from build123d import *

# Parameters (mm, degrees)
BOSS_EXTRUDE1_DEPTH = 10
SKETCH2_R           = 1
BOSS_EXTRUDE2_DEPTH = 2.25


with BuildPart() as part:
    # Sketch1 → Boss-Extrude1 (new body)
    with BuildSketch(Plane(origin=(0, 0, 0), x_dir=(1, 0, 0), z_dir=(0, 1, 0))):
        with BuildLine():
            ThreePointArc((-0.855605783, -5.938681566), (-6, 0), (-0.855605783, 5.938681566))
            Line((-0.855605783, 5.938681566), (-1.283408674, 8.908022349))
            ThreePointArc((-1.283408674, 8.908022349), (-9, 0), (-1.283408674, -8.908022349))
            Line((-1.283408674, -8.908022349), (-0.855605783, -5.938681566))
        make_face()
    extrude(amount=BOSS_EXTRUDE1_DEPTH)

    # Sketch2 → Boss-Extrude2 (add)
    with BuildSketch(Plane(origin=(0, 10, 0), x_dir=(1, 0, 0), z_dir=(0, 1, 0))):
        with Locations(Location((-7.5, 0, 0), (0, 0, 270))):
            Circle(SKETCH2_R)
    extrude(amount=BOSS_EXTRUDE2_DEPTH)


solid = part.part
The listing builds one solid part. Answer for the finished solid, in the listing's coordinates (mm). A direction names the side the tool comes from. Give positions to 0.01 mm unless a question says otherwise; leave off trailing zeros. Write each loop counter-clockwise with the first axis right and the second up, starting at its lowest first coordinate (ties: lowest second). Pieces come first, ordered by that corner, then holes.
1) Section C-C (x = -7.75) is taken. Write down the section's boundary in (y, z), and give its area (3 significant figures).
2) Section A-A (x = -3) is taken. Write down the section's boundary in (y, z), and give its area (3 significant figures).
3) For a pull along Z with two mould halves and no side action, classify faces 1 (the face through (-7, 12.25, 0)), 2 (the face through (-1.067, 4.93, -7.403)), 3 (the face through (-6, 5, 0)) as pulls with the +Z half, pulls with the -Z half, needs draft (parallel to the pull), parting line crosses it, or undercut.
4) Given P1, Ø3, axis at x = -5, y = 5.5, coming from the -Z side, flat-ended and moving along its own axis, determine where the tip first touches the part or whether it passes through.
5) Section D-D (y = 7.25) is taken. Write down the section's boundary in (x, z).
6) Section B-B (z = 0) is taken. Write down the section's boundary in (x, y), and give its area (3 significant figures).
7) Find the intervals of material crossed by L1, parallel to Y at x = -3.5, z = 7.25; L2, parallel to Z at x = -5.5, y = 6; L3, parallel to Z at x = -1.75, y = 5.25, in increasing order.
8) A tool of negligible diameter and unlimited length cuts with its end or side. For faces 4 (the face through (-6.51, 11.11, -0.13)), 5 (the face through (-7, 0, 0)), from which of +Z, -Z, +X, -X, +Y, -Y can it reach the whole face along a straight path? Write none if from no direction.
Response:
1. outline: (0, -4.58) - (10, -4.58) - (10, -0.97) - (12.25, -0.97) - (12.25, 0.97) - (10, 0.97) - (10, 4.58) - (0, 4.58) - close
1. area: 95.9 mm2
2. outline: (0, -8.49) - (10, -8.49) - (10, -5.2) - (0, -5.2) - close; (0, 5.2) - (10, 5.2) - (10, 8.49) - (0, 8.49) - close
2. area: 65.8 mm2
3. face 1: needs draft
3. face 2: pulls with the -Z half
3. face 3: undercut
4. P1: stops at z = -8.29
5. outline: (-1.28, -8.91) - (-0.86, -5.94) arc R6 cw to (-0.86, 5.94) - (-1.28, 8.91) arc R9 ccw to start
6. outline: (-9, 0) - (-6, 0) - (-6, 10) - (-6.5, 10) - (-6.5, 12.25) - (-8.5, 12.25) - (-8.5, 10) - (-9, 10) - close
6. area: 34.5 mm2
7. L1: y = 0 to 10
7. L2: z = -7.12 to -2.4, 2.4 to 7.12
7. L3: z = -8.83 to -5.74, 5.74 to 8.83
8. face 4: +Y
8. face 5: +Z, -Z, +X, -X, -Y
